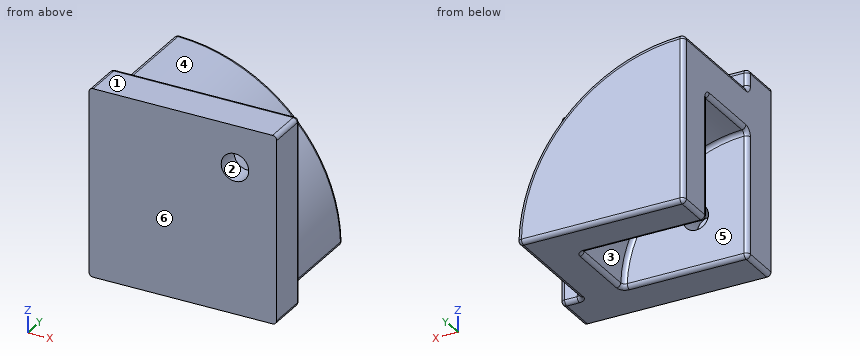
from build123d import *

# Parameters (mm, degrees)
SKETCH3_W                               = 45
SKETCH3_H                               = 45
BOSS_EXTRUDE1_DEPTH                     = 10
CBORE_FOR_M6_HEX_HEAD_BOLT1_D           = 6.6
CBORE_FOR_M6_HEX_HEAD_BOLT1_CBORE_D     = 14.55
CBORE_FOR_M6_HEX_HEAD_BOLT1_CBORE_DEPTH = 4.38
BOSS_EXTRUDE3_DEPTH                     = 18
BOSS_EXTRUDE4_DEPTH                     = 10
SKETCH10_R                              = 3
CUT_EXTRUDE2_DEPTH                      = 6
FILLET2_R                               = 1


with BuildPart() as part:
    # Sketch3 → Boss-Extrude1 (new body)
    with BuildSketch(Plane(origin=(0, 0, 0), x_dir=(1, 0, 0), z_dir=(0, 1, 0))):
        Rectangle(SKETCH3_W, SKETCH3_H)
    extrude(amount=BOSS_EXTRUDE1_DEPTH)

    # CBORE for M6 Hex Head Bolt1 (through all)
    with Locations(Plane(origin=(0, 10, 0), x_dir=(1, 0, 0), z_dir=(0, 1, 0))):
        with Locations((12.5, -12.5)):
            CounterBoreHole(CBORE_FOR_M6_HEX_HEAD_BOLT1_D / 2, CBORE_FOR_M6_HEX_HEAD_BOLT1_CBORE_D / 2, CBORE_FOR_M6_HEX_HEAD_BOLT1_CBORE_DEPTH)

    # Sketch8 → Boss-Extrude3 (add)
    with BuildSketch(Plane(origin=(0, 10, 0), x_dir=(1, 0, 0), z_dir=(0, 1, 0))):
        with BuildLine():
            Line((17.5, 22.5), (7.5, 22.5))
            ThreePointArc((7.5, 22.5), (-1.286796564, 1.286796564), (-22.5, -7.5))
            Line((-22.5, -7.5), (-22.5, -17.5))
            ThreePointArc((-22.5, -17.5), (5.784271247, -5.784271247), (17.5, 22.5))
        make_face()
    extrude(amount=BOSS_EXTRUDE3_DEPTH)

    # Sketch9 → Boss-Extrude4 (add)
    with BuildSketch(Plane(origin=(0, 28, 0), x_dir=(1, 0, 0), z_dir=(0, 1, 0))):
        with BuildLine():
            Line((17.5, 22.5), (-22.5, 22.5))
            Line((-22.5, 22.5), (-22.5, -17.5))
            ThreePointArc((-22.5, -17.5), (5.784271247, -5.784271247), (17.5, 22.5))
        make_face()
    extrude(amount=BOSS_EXTRUDE4_DEPTH)

    # Sketch10 → Cut-Extrude2 (cut)
    with BuildSketch(Plane(origin=(0, 10, 0), x_dir=(1, 0, 0), z_dir=(0, 1, 0))):
        with Locations(Location((-10, 10, 0), (0, 0, 270))):
            Circle(SKETCH10_R)
    extrude(amount=-CUT_EXTRUDE2_DEPTH, mode=Mode.SUBTRACT)

    # Fillet2
    fillet2_edges = [part.edges().sort_by_distance(p)[0] for p in [
        (-22.5, 10, -7.5),
        (0, 10, 22.5),
        (-7.5, 10, -22.5),
        (-22.5, 10, 20),
        (5.784271247, 10, 5.784271247),
        (-22.5, 24, 17.5),
        (17.5, 24, -22.5),
        (-1.286796564, 10, -1.286796564),
        (7.5, 19, -22.5),
        (-22.5, 19, 7.5),
        (-1.286796564, 28, -1.286796564),
        (-22.5, 28, -7.5),
        (-22.5, 33, -22.5),
        (-7.5, 28, -22.5),
        (-22.5, 38, -2.5),
        (5.784271247, 38, 5.784271247),
        (-2.5, 38, -22.5),
        (22.5, 10, 0),
        (22.5, 5, 22.5),
        (-22.5, 5, 22.5),
        (-22.5, 5, -22.5),
        (22.5, 5, -22.5),
        (20, 10, -22.5),
    ]]
    fillet(fillet2_edges, radius=FILLET2_R)


solid = part.part
The model under review builds one solid part; all positions refer to its coordinate system, in mm. Face numbers are marked on the shaded views. A direction names the side the tool comes from. Round coordinates to 2 decimals unless told otherwise and drop trailing zeros. Loops run counter-clockwise (first coordinate to the right, second up) from the corner with the lowest first, then second, coordinate; pieces in that order, holes last. Notation, with made-up numbers: (88, 85.25) -> (99, 85.25) arc R25 ccw to (99, 108.25) -> close; hole circle Ø1 at (-16, 10.25). An arc over 180 degrees is marked (long way). Answer as CSV lines item,"result".
1) Tool access review of the marked faces 4, 5 and 6: name each direction out of +Z, -Z, +X, -X, +Y, -Y from which nothing blocks a thin tool from reaching the whole face with its end or side.
Geometry results:
face 4,"+Z, +X, +Y"
face 5,"-Z, -X"
face 6,"+Z, -Z, +X, -X, -Y"
2) Add section B-B on y = 34.5. Write out the cut boundary in (x, z), plus the area to 3 significant figures.
Geometry results:
outline,"(-22.5, -21.5) arc R1 ccw to (-21.5, -22.5) -> (16.49, -22.5) arc R1 ccw to (17.49, -21.47) arc R40 ccw to (-21.47, 17.49) arc R1 ccw to (-22.5, 16.49) -> close"
area,"1,260 mm²"
3) Draft analysis for pull direction Z (two halves, no side actions). For the marked faces 1, 2 and 3, state which applies: pulls with the +Z half, pulls with the -Z half, needs draft (parallel to the pull), parting line crosses it, or undercut.
Geometry results:
face 1,"pulls with the +Z half"
face 2,"undercut"
face 3,"pulls with the -Z half"
4) Add section A-A on y = 23.5. Write out the cut boundary in (x, z).
Geometry results:
outline,"(-22.5, 8.48) arc R1 ccw to (-21.53, 7.48) arc R30 cw to (7.48, -21.53) arc R1 ccw to (8.48, -22.5) -> (16.49, -22.5) arc R1 ccw to (17.49, -21.47) arc R40 ccw to (-21.47, 17.49) arc R1 ccw to (-22.5, 16.49) -> close"
5) To check wall thickness, follow line 1 along Y through (x, z) = (-12, -10.5); line 2 along Z through (x, y) = (12.5, 7.8) (3 decimals); line 3 along Y through (x, z) = (-12, 4.5). State the ranges of each line that lie inside material, in increasing order. Write a range as from..to.
Geometry results:
line 1,"y = 0..4, 28..38"
line 2,"z = -22.5..5.225, 19.775..22.5"
line 3,"y = 0..10, 28..38"
6) For P1, Ø1.5, axis at x = 6, z = 10.5, coming from the +Y side; P2, Ø1.5, axis at x = 15, z = 7, coming from the +Y side; P3, Ø6, axis at x = 12.5, z = 12.5, coming from the -Y side; P4, Ø1.5, axis at y = 23.5, z = -15.5, coming from the +X side, all flat-tipped, find the tip position at first contact; note any pin that passes through.
Geometry results:
P1,"stops at y = 10"
P2,"stops at y = 5.62"
P3,"passes through"
P4,"stops at x = 17.01"
